Design review of the part built by this model. Coordinates are the model's own, in mm. Face numbers are marked on the shaded views. A direction names the side the tool comes from. Coordinates: 2 decimals unless noted, no trailing zeros. Write each loop counter-clockwise with the first axis right and the second up, starting at its lowest first coordinate (ties: lowest second). Pieces come first, ordered by that corner, then holes. Notation, with made-up numbers: (70, 19.25) - (115, 19.25) arc R24 ccw to (115, 50.25) - close; hole circle Ø8 at (12, 69). An arc over 180 degrees is marked (long way). Answer as a JSON object with one key per item and string values.
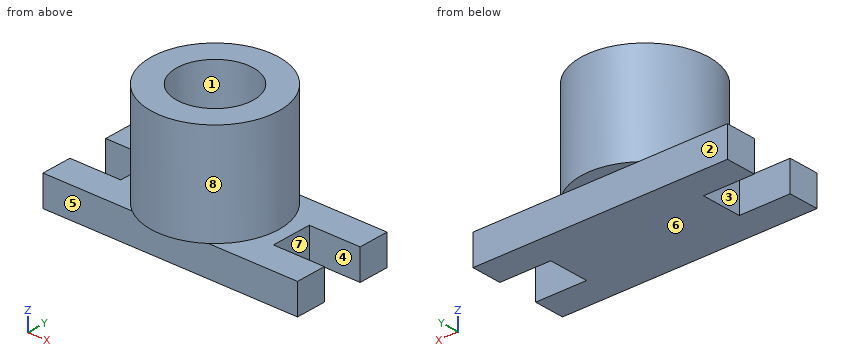
```python
from build123d import *

# Parameters (mm, degrees)
F0_W     = 100
F0_H     = 40
F1_DEPTH = 12
F2_W     = 20
F2_H     = 16
F3_DEPTH = 12.001
F4_R     = 25
F5_DEPTH = 40
F6_R     = 15
F7_DEPTH = 20


with BuildPart() as f1:
    # F0 (on Top) → F1 (new body)
    with BuildSketch(Plane.XY):
        Rectangle(F0_W, F0_H)
    extrude(amount=F1_DEPTH)

    # F2 (on face) → F3 (cut, through all)
    with BuildSketch(Plane.XY.offset(12)):
        with Locations((-40, 0)):
            Rectangle(F2_W, F2_H)
        with Locations((40, 0)):
            Rectangle(F2_W, F2_H)
    extrude(amount=-F3_DEPTH, mode=Mode.SUBTRACT)

    # F4 (on face) → F5 (join)
    with BuildSketch(Plane.XY.offset(12)):
        Circle(F4_R)
    extrude(amount=F5_DEPTH)

    # F6 (on face) → F7 (cut)
    with BuildSketch(Plane.XY.offset(52)):
        Circle(F6_R)
    extrude(amount=-F7_DEPTH, mode=Mode.SUBTRACT)


solid = f1.part
```
(1) To check wall thickness, follow line 1 (Y direction, x = 0, z = 46.5); line 2 (X direction, y = 1, z = 19.5); line 3 (Z direction, x = -33, y = -13). State the ranges of each line that lie inside material, in increasing order. Write a range as from..to.
Solved:
{"line 1": "y = -25..-15, 15..25", "line 2": "x = -24.98..24.98", "line 3": "z = 0..12"}
(2) Take a section at B-B, the plane z = 41.5. Write out the cut boundary in (x, y).
Solved:
{"outline": "circle Ø50 at (0, 0); hole circle Ø30 at (0, 0)"}
(3) Take a section at C-C, the plane y = 0. Write out the cut boundary in (x, z), and give its area (3 significant figures).
Solved:
{"outline": "(-30, 0) - (30, 0) - (30, 12) - (25, 12) - (25, 52) - (15, 52) - (15, 32) - (-15, 32) - (-15, 52) - (-25, 52) - (-25, 12) - (-30, 12) - close", "area": "2,120 mm^2"}
(4) The part is to be moulded in two halves that separate along Y. For the marked faces 5, 6, 7 and 8, say which applies: pulls with the +Y half, pulls with the -Y half, needs draft (parallel to the pull), parting line crosses it, or undercut.
Solved:
{"face 5": "pulls with the -Y half", "face 6": "needs draft", "face 7": "undercut", "face 8": "parting line crosses it"}
(5) Tool access review of the marked faces 1, 2, 3 and 4: name each direction out of +Z, -Z, +X, -X, +Y, -Y from which nothing blocks a thin tool from reaching the whole face with its end or side.
Solved:
{"face 1": "+Z", "face 2": "-Z, +X, -X, +Y", "face 3": "+Z, -Z, -X", "face 4": "+Z, -Z, +X"}
(6) Take a section at A-A, the plane x = 0. Write out the cut boundary in (y, z), and give its area (3 significant figures).
Solved:
{"outline": "(-25, 12) - (-20, 12) - (-20, 0) - (20, 0) - (20, 12) - (25, 12) - (25, 52) - (15, 52) - (15, 32) - (-15, 32) - (-15, 52) - (-25, 52) - close", "area": "1,880 mm^2"}
(7) For pin 1 (3.5 mm diameter, centred on y = 3.5, z = 4.5, fed in from +X); pin 2 (3.5 mm diameter, centred on x = 41, z = 6, fed in from +Y); pin 3 (4 mm diameter, centred on x = 6, y = -22.5, fed in from -Z); pin 4 (8 mm diameter, centred on x = 30, z = 35.5, fed in from +Y), all flat-tipped, find the tip position at first contact; note any pin that passes through.
Solved:
{"pin 1": "stops at x = 30", "pin 2": "stops at y = 20", "pin 3": "stops at z = 12", "pin 4": "passes through"}
(8) Take a section at D-D, the plane z = 31. Write out the cut boundary in (x, y).
Solved:
{"outline": "circle Ø50 at (0, 0)"}
